Input: part model. Units: mm. Frame: model coordinates. A direction names the side the tool comes from. Give positions to 0.01 mm unless a question says otherwise; leave off trailing zeros. Order: outer loops, then holes, each group sorted by start corner. A loop starts at its lowest first (then second) coordinate and runs counter-clockwise, first axis right, second up. Notation, with made-up numbers: (-20.75, 58.25) -> (13.25, 58.25) arc R25 cw to (13.25, 73.25) -> close; hole circle Ø1 at (-1.5, 79). An arc over 180 degrees is marked (long way). Use a Markdown table: item, result. Add a question column.
from build123d import *

# Parameters (mm, degrees)
F1_DEPTH = 9
F0_R     = 1.5
F2_DEPTH = 6


# Not quite as in the source:
# - a feature names something its author has since deleted; it is built from what else it names


with BuildPart() as f1:
    # F0 (on Right) → F1 (new body)
    with BuildSketch(Plane.YZ):
        with BuildLine():
            Line((0, 115), (-67.5, 115))
            Line((-67.5, 115), (-67.5, -115))
            Line((-67.5, -115), (0, -115))
            Line((0, -115), (0, -70.25))
            ThreePointArc((0, -70.25), (-37.75, -32.5), (0, 5.25))
            Line((0, 5.25), (0, 51))
            ThreePointArc((0, 51), (-22, 73), (0, 95))
            Line((0, 95), (0, 115))
        make_face()
        with BuildLine():
            Line((67.5, 115), (0, 115))
            Line((0, 115), (0, 95))
            ThreePointArc((0, 95), (15.5563491861, 88.5563491861), (22, 73))
            ThreePointArc((22, 73), (15.5563491861, 57.4436508139), (0, 51))
            Line((0, 51), (0, 5.25))
            ThreePointArc((0, 5.25), (26.6932809898, -5.8067190102), (37.75, -32.5))
            ThreePointArc((37.75, -32.5), (26.6932809898, -59.1932809898), (0, -70.25))
            Line((0, -70.25), (0, -115))
            Line((0, -115), (67.5, -115))
            Line((67.5, -115), (67.5, 115))
        make_face()
    extrude(amount=F1_DEPTH)

    # F0 (on Right) → F2 (join)
    with BuildSketch(Plane.YZ):
        with BuildLine():
            Line((0, 89.5), (0, 95))
            ThreePointArc((0, 95), (-22, 73), (0, 51))
            Line((0, 51), (0, 56.5))
            ThreePointArc((0, 56.5), (-16.5, 73), (0, 89.5))
        make_face()
        with BuildLine():
            ThreePointArc((22, 73), (15.5563491861, 88.5563491861), (0, 95))
            Line((0, 95), (0, 89.5))
            ThreePointArc((0, 89.5), (11.6672618896, 84.6672618896), (16.5, 73))
            ThreePointArc((16.5, 73), (11.6672618896, 61.3327381104), (0, 56.5))
            Line((0, 56.5), (0, 51))
            ThreePointArc((0, 51), (15.5563491861, 57.4436508139), (22, 73))
        make_face()
        with BuildLine():
            ThreePointArc((0, 5.25), (-37.75, -32.5), (0, -70.25))
            Line((0, -70.25), (0, -55.25))
            ThreePointArc((0, -55.25), (-22.75, -32.5), (0, -9.75))
            Line((0, -9.75), (0, 5.25))
        make_face()
        with Locations((-21.5667568262, -54.0667568262)):
            Circle(F0_R, mode=Mode.SUBTRACT)
        with Locations((-21.5667568262, -10.9332431738)):
            Circle(F0_R, mode=Mode.SUBTRACT)
        with BuildLine():
            Line((0, -55.25), (0, -70.25))
            ThreePointArc((0, -70.25), (26.6932809898, -59.1932809898), (37.75, -32.5))
            ThreePointArc((37.75, -32.5), (26.6932809898, -5.8067190102), (0, 5.25))
            Line((0, 5.25), (0, -9.75))
            ThreePointArc((0, -9.75), (16.086679272, -16.413320728), (22.75, -32.5))
            ThreePointArc((22.75, -32.5), (16.086679272, -48.586679272), (0, -55.25))
        make_face()
        with Locations((21.5667568262, -54.0667568262)):
            Circle(F0_R, mode=Mode.SUBTRACT)
        with Locations((21.5667568262, -10.9332431738)):
            Circle(F0_R, mode=Mode.SUBTRACT)
    extrude(amount=F2_DEPTH)


solid = f1.part
Q1. Section query D-D (z = -64.5). Return loops of the section in (x, y).
Q2. Draft query along Z for faces 1 (the cylindrical face through (7.48, 20.32, 81.43)), 2 (the flat face through (4, -1, -115)), 3 (the flat face through (4, 67.5, -2)). Return one class per face: +Z half, -Z half, draft (parallel to the pull), parting line (faces both ways), or undercut.
Q3. Section query C-C (y = -14). Return loops of the section in (x, z).
Q4. First-contact query: pin 1 (5 mm diameter, centred on y = -21.57, z = -54.07, fed in from -X); pin 2 (2.5 mm diameter, centred on y = -21.57, z = -10.93, fed in from +X); pin 3 (22.5 mm diameter, centred on y = -3, z = -20.5, fed in from +X). Flat tips, straight axial feed; report the tip coordinate or a pass-through.
Q5. Section query A-A (z = -32.5). Return loops of the section in (x, y), plus the area to 4 significant figures.
Q6. Access query for faces 4 (the flat face through (6, 16, -49)), 5 (the cylindrical face through (2.958, -18.054, -18.657)). Directions: +Z, -Z, +X, -X, +Y, -Y. A direction counts if a zero-diameter tool reaches every point of the face in a straight line with its end or side. Return the directions, or none.
Q7. Section query B-B (x = 2.75). Return loops of the section in (y, z).
Q8. Ray query, line 1 (Z direction, x = 7, y = 0); line 2 (Y direction, x = 4.5, z = 72); line 3 (Y direction, x = 3.75, z = -32.5). Return the intervals inside material, ascending.
Solution:
| question | item | result |
|---|---|---|
| 1 | outline | (0, -67.5) -> (9, -67.5) -> (9, -20.03) -> (6, -20.03) -> (6, 20.03) -> (9, 20.03) -> (9, 67.5) -> (0, 67.5) -> close |
| 2 | face 1 | undercut |
| 2 | face 2 | -Z half |
| 2 | face 3 | draft |
| 3 | outline | (0, -115) -> (9, -115) -> (9, -67.56) -> (6, -67.56) -> (6, -50.43) -> (0, -50.43) -> close; (0, -14.57) -> (6, -14.57) -> (6, 2.56) -> (9, 2.56) -> (9, 56.03) -> (6, 56.03) -> (6, 64.27) -> (0, 64.27) -> close; (0, 81.73) -> (6, 81.73) -> (6, 89.97) -> (9, 89.97) -> (9, 115) -> (0, 115) -> close |
| 4 | pin 1 | stops at x = 0 |
| 4 | pin 2 | passes through |
| 4 | pin 3 | stops at x = 6 |
| 5 | outline | (0, -67.5) -> (9, -67.5) -> (9, -37.75) -> (6, -37.75) -> (6, -22.75) -> (0, -22.75) -> close; (0, 22.75) -> (6, 22.75) -> (6, 37.75) -> (9, 37.75) -> (9, 67.5) -> (0, 67.5) -> close |
| 5 | area | 715.5 mm² |
| 6 | face 4 | +X |
| 6 | face 5 | +X, -X |
| 7 | outline | (-67.5, -115) -> (67.5, -115) -> (67.5, 115) -> (-67.5, 115) -> close; hole circle Ø3 at (-21.57, -54.07); hole circle Ø3 at (-21.57, -10.93); hole circle Ø45.5 at (0, -32.5); hole circle Ø33 at (0, 73); hole circle Ø3 at (21.57, -54.07); hole circle Ø3 at (21.57, -10.93) |
| 8 | line 1 | z = -115 to -70.25, 5.25 to 51, 95 to 115 |
| 8 | line 2 | y = -67.5 to -16.47, 16.47 to 67.5 |
| 8 | line 3 | y = -67.5 to -22.75, 22.75 to 67.5 |
